```python
from build123d import *

# Parameters (mm, degrees)
EXTRUSION1_DEPTH             = 2
ESQUISSE2_R                  = 3
EXTRUSION2_DEPTH             = 6
ESQUISSE3_R                  = 3.05
EXTRUSION3_DEPTH             = 1
ENL_V_MAT_EXTRU_1_DEPTH      = 17.450303949
ENL_V_MAT_EXTRU_1_DEPTH_BACK = 17.450303949
ESQUISSE4_R                  = 1.5


with BuildPart() as part:
    # Esquisse1 → Extrusion1 (new body)
    with BuildSketch(Plane.XY):
        with BuildLine():
            Line((3, 0), (11, 0))
            ThreePointArc((11, 0), (13.121320344, 0.878679656), (14, 3))
            Line((14, 3), (14, 3.1))
            ThreePointArc((14, 3.1), (13.121320344, 5.221320344), (11, 6.1))
            Line((11, 6.1), (3, 6.1))
            ThreePointArc((3, 6.1), (0.878679656, 5.221320344), (0, 3.1))
            Line((0, 3.1), (0, 3))
            ThreePointArc((0, 3), (0.878679656, 0.878679656), (3, 0))
        make_face()
    extrude(amount=EXTRUSION1_DEPTH)

    # Esquisse2 → Extrusion2 (add)
    with BuildSketch(Plane.XY.offset(2)):
        with Locations(Location((3, 3.05, 0), (0, 0, 180))):
            Circle(ESQUISSE2_R)
    extrude(amount=EXTRUSION2_DEPTH)

    # Esquisse3 → Extrusion3 (add)
    with BuildSketch(Plane(origin=(0, 0, 0), x_dir=(-1, 0, 0), z_dir=(0, 0, -1))):
        with Locations(Location((-11, 3.05, 0), (0, 0, 270))):
            Circle(ESQUISSE3_R)
    extrude(amount=EXTRUSION3_DEPTH)

    # Esquisse4 → Enlèv. mat.-Extru.1 (cut, two sides: drawn at the far end of the back side and taken through both)
    with BuildSketch(Plane.XY.offset(2).offset(-ENL_V_MAT_EXTRU_1_DEPTH_BACK)):
        with Locations((3, 3.05)):
            Circle(ESQUISSE4_R)
        with Locations((11, 3.05)):
            Circle(ESQUISSE4_R)
    extrude(amount=ENL_V_MAT_EXTRU_1_DEPTH + ENL_V_MAT_EXTRU_1_DEPTH_BACK, mode=Mode.SUBTRACT)


solid = part.part
```
CAD build for the part. Positions are in the model's coordinates, mm. A direction names the side the tool comes from. Coordinates: 2 decimals unless noted, no trailing zeros. Order: outer loops, then holes, each group sorted by start corner. A loop starts at its lowest first (then second) coordinate and runs counter-clockwise, first axis right, second up.
(1) Which spindle directions (+Z, -Z, +X, -X, +Y, -Y) get a long thin tool onto all of the face, cutting with end or side? Do faces 1 (the face through (7.976, 3.447, -0.493)), 2 (the face through (0.9, 5.24, 0.99)), 3 (the face through (13.14, 5.2, 0.99)), 4 (the face through (4.386, 2.475, 3.944)), 5 (the face through (13.1, 0.86, 0.99)). Say none if no direction does.
Solution:
face 1: -Z
face 2: +Z, -Z, -X, +Y
face 3: +Z, +X, +Y
face 4: +Z, -Z
face 5: +Z, +X, -Y
(2) Pin check, flat tips, straight feed: pin 1 Ø3 at (x, y) = (5.5, 3) entering from -Z; pin 2 Ø1 at (y, z) = (5.5, 1) entering from -X; pin 3 Ø4 at (x, z) = (4.5, 5) entering from +Y. Stop position of each tip, or through.
Solution:
pin 1: stops at z = 0
pin 2: stops at x = 0.68
pin 3: stops at y = 6.05
(3) Saw through at A-A, the plane z = 1.25. Write the cut outline in (x, y), and give its area (3 significant figures).
Solution:
outline: (0, 3) arc R3 ccw to (3, 0) - (11, 0) arc R3 ccw to (14, 3) - (14, 3.1) arc R3 ccw to (11, 6.1) - (3, 6.1) arc R3 ccw to (0, 3.1) - close; hole circle Ø3 at (3, 3.05); hole circle Ø3 at (11, 3.05)
area: 63.5 mm2
(4) Saw through at C-C, the plane y = 3.25. Count the separate pieces of the cut face and the enclosed holes in it, and give its area (3 significant figures).
Solution:
separate pieces: 3
enclosed holes: 0
area: 37.3 mm2
(5) Saw through at B-B, the plane x = 10. Write the cut outline in (y, z).
Solution:
outline: (0, 0) - (0.17, 0) - (0.17, -1) - (1.93, -1) - (1.93, 2) - (0, 2) - close; (4.17, -1) - (5.93, -1) - (5.93, 0) - (6.1, 0) - (6.1, 2) - (4.17, 2) - close
(6) Saw through at D-D, the plane z = 6. Write the cut outline in (x, y).
Solution:
outline: circle Ø6 at (3, 3.05); hole circle Ø3 at (3, 3.05)
(7) Mould opens along X. For faces 6 (the face through (5.21, 1.02, 4.96)), 7 (the face through (9.5, 3.1, 0.5)), 8 (the face through (5, 3, 0)) say: released by +X, released by -X, zero draft, split by the parting line, or undercut.
Solution:
face 6: split by the parting line
face 7: undercut
face 8: zero draft
(8) Drill centre lines: L1, parallel to X at y = 3.05, z = 0.6; L2, parallel to Y at x = 3, z = 5; L3, parallel to X at y = 2.5, z = 1.25. Where is each one in solid material? Low to high.
Solution:
L1: x = 0 to 1.5, 4.5 to 9.5, 12.5 to 14
L2: y = 0.05 to 1.55, 4.55 to 6.05
L3: x = 0.04 to 1.6, 4.4 to 9.6, 12.4 to 13.96
